Geometry: final body of the model. Coordinates: model frame, mm. A direction names the side the tool comes from. Round coordinates to 2 decimals unless told otherwise and drop trailing zeros. Write each loop counter-clockwise with the first axis right and the second up, starting at its lowest first coordinate (ties: lowest second). Pieces come first, ordered by that corner, then holes.
from build123d import *

# Parameters (mm, degrees)
BOSS_EXTRUDE1_DEPTH   = 9.525
SKETCH6_R             = 4.800000000000002
CUT_EXTRUDE1_DEPTH    = 57.261143340675204
SKETCH10_R            = 2.2859999999999947
CUT_EXTRUDE2_DEPTH    = 3.8099999999999996
F_8_CLEARANCE_HOLE1_D = 4.4958
SKETCH13_W            = 109.6136957213275
SKETCH13_H            = 27.196963560799638
CUT_EXTRUDE3_DEPTH    = 57.261143340675204
CUT_EXTRUDE5_DEPTH    = 57.2611433406752
FILLET1_R             = 2.54
SKETCH15_R            = 2.24789999999999
CUT_EXTRUDE6_DEPTH    = 57.26114334073907


with BuildPart() as part:
    # Sketch1 → Boss-Extrude1 (new body)
    with BuildSketch(Plane.XY):
        Polygon((50.79999999999998, -22.225), (-50.800000000000004, -22.225000000000012), (-50.800000000000004, 22.224999999999984), (50.79999999999999, 22.224999999999998), align=None)
    extrude(amount=BOSS_EXTRUDE1_DEPTH)

    # Sketch6 → Cut-Extrude1 (cut, through all)
    with BuildSketch(Plane.XY):
        with Locations(Location((-25.4, 9.524999999999999, 0), (0, 0, 180))):
            Circle(SKETCH6_R)
    extrude(amount=CUT_EXTRUDE1_DEPTH, mode=Mode.SUBTRACT)

    # Sketch10 → Cut-Extrude2 (cut)
    with BuildSketch(Plane.XY.offset(9.525)):
        with Locations((-46.11545283004946, -16.76399999999999)):
            Circle(SKETCH10_R)
    extrude(amount=-CUT_EXTRUDE2_DEPTH, mode=Mode.SUBTRACT)

    # #8 Clearance Hole1 (through all)
    with Locations(Plane(origin=(0, 0, 0), x_dir=(-1, 0, 0), z_dir=(0, 0, -1))):
        with Locations((-43.931814057, 8.51848178), (-31.231814057, 8.51848178)):
            Hole(F_8_CLEARANCE_HOLE1_D / 2)

    # Sketch13 → Cut-Extrude3 (cut, through all)
    with BuildSketch(Plane(origin=(0, 0, 0), x_dir=(-1, 0, 0), z_dir=(0, 0, -1))):
        with Locations((0, -22.225000000072345)):
            Rectangle(SKETCH13_W, SKETCH13_H)
    extrude(amount=-CUT_EXTRUDE3_DEPTH, mode=Mode.SUBTRACT)

    # Sketch14 → Cut-Extrude5 (cut, through all)
    with BuildSketch(Plane(origin=(0, 0, 0), x_dir=(-1, 0, 0), z_dir=(0, 0, -1))):
        Polygon((-50.80000000007075, 14.368885078592964), (-1.0960952551413707, 14.368885078592964), (-0.33859307620571544, 15.218043280381785), (6.4513217163673575, 22.82952215911174), (6.4513217163673575, 26.369267610296045), (-61.117569834071936, 26.369267610296045), (-61.117569834071936, 13.29236417327235), align=None)
    extrude(amount=-CUT_EXTRUDE5_DEPTH, mode=Mode.SUBTRACT)

    # Fillet1
    fillet1_edges = [part.edges().sort_by_distance(p)[0] for p in [
        (-5.912050174530525, 22.22499999999999, 4.7625),
        (1.0960952551413707, 14.368885078592964, 4.7625),
    ]]
    fillet(fillet1_edges, radius=FILLET1_R)

    # Sketch15 → Cut-Extrude6 (cut, through all)
    with BuildSketch(Plane(origin=(0, 0, 0), x_dir=(-1, 0, 0), z_dir=(0, 0, -1))):
        with Locations((44.4499999999996, 8.139974193482002)):
            Circle(SKETCH15_R)
    extrude(amount=-CUT_EXTRUDE6_DEPTH, mode=Mode.SUBTRACT)


solid = part.part
1) Section B-B on z = 7.75. Output: boundary loops of the cut face in (x, y) (3 decimals), plus the area to 3 significant figures.
2) First-contact query: P1, Ø4, axis at x = -44.45, y = 8.14, coming from the +Z side. Flat tip, straight axial feed; report the tip coordinate or a pass-through.
3) Section A-A on x = -44.45. Output: boundary loops of the cut face in (y, z) (3 decimals), plus the area to 3 significant figures.
4) Draft query along X for faces 3 (the flat face through (1, 4, 9.525)), 4 (the cylindrical face through (1.209, 14.585, 4.829)), 5 (the cylindrical face through (33.376, 9.194, 4.829)). Return one class per face: pulls with the +X half, pulls with the -X half, needs draft (parallel to the pull), parting line crosses it, or undercut.
5) Line query: probe 1 along X at (y, z) = (8.5, 4.5); probe 2 along Y at (x, z) = (-44.45, 2) (3 decimals); probe 3 along X at (y, z) = (7.5, 1.5). Output: solid intervals per line, ascending.
6) Section C-C on x = -25.4. Output: boundary loops of the cut face in (y, z) (3 decimals).
7) Reachability of faces 1 (the flat face through (27, 14.369, 5)), 2 (the flat face through (1, -8.627, 5)) from +Z, -Z, +X, -X, +Y, -Y: full face, straight path, thin tool, end or side. Return the list, or none.
Filled in:
1. outline: (-50.8, -8.627) - (50.8, -8.627) - (50.8, 14.369) - (2.234, 14.369) arc R2.54 cw to (0.339, 15.218) - (-5.155, 21.376) arc R2.54 ccw to (-7.05, 22.225) - (-50.8, 22.225) - close; hole circle Ø4.496 at (-44.45, 8.14); hole circle Ø9.6 at (-25.4, 9.525); hole circle Ø4.496 at (31.232, 8.518); hole circle Ø4.496 at (43.932, 8.518)
1. area: 2,600 mm2
2. P1: passes through
3. outline: (-8.627, 0) - (5.892, 0) - (5.892, 9.525) - (-8.627, 9.525) - close; (10.388, 0) - (22.225, 0) - (22.225, 9.525) - (10.388, 9.525) - close
3. area: 251 mm2
4. face 3: needs draft
4. face 4: pulls with the +X half
4. face 5: undercut
5. probe 1: x = -50.8 to -46.67, -42.23 to -30.09, -20.71 to 28.98, 33.48 to 41.68, 46.18 to 50.8
5. probe 2: y = -8.627 to 5.892, 10.388 to 22.225
5. probe 3: x = -50.8 to -46.6, -42.3 to -29.75, -21.05 to 29.23, 33.24 to 41.93, 45.94 to 50.8
6. outline: (-8.627, 0) - (4.725, 0) - (4.725, 9.525) - (-8.627, 9.525) - close; (14.325, 0) - (22.225, 0) - (22.225, 9.525) - (14.325, 9.525) - close
7. face 1: +Z, -Z, +X, +Y
7. face 2: +Z, -Z, +X, -X, -Y
